```python
from build123d import *


with BuildPart() as f1:
    # F0 (on Front) → F1 (revolve)
    with BuildSketch(Plane.XZ):
        with BuildLine():
            Line((0, 201.6125), (0, 114.3))
            Line((0, 114.3), (0, 26.9875))
            ThreePointArc((0, 26.9875), (1.5875, 25.4), (3.175, 26.9875))
            Line((3.175, 26.9875), (3.175, 28.575))
            Line((3.175, 28.575), (2.159, 28.575))
            Line((2.159, 28.575), (2.159, 31.75))
            Line((2.159, 31.75), (3.175, 31.75))
            Line((3.175, 31.75), (3.175, 114.3))
            Line((3.175, 114.3), (3.175, 196.85))
            Line((3.175, 196.85), (2.159, 196.85))
            Line((2.159, 196.85), (2.159, 200.025))
            Line((2.159, 200.025), (3.175, 200.025))
            Line((3.175, 200.025), (3.175, 201.6125))
            ThreePointArc((3.175, 201.6125), (1.5875, 203.2), (0, 201.6125))
        make_face()
    revolve(axis=Axis((15.875, 0, 158.75), (0, 0, -1)))


solid = f1.part
```
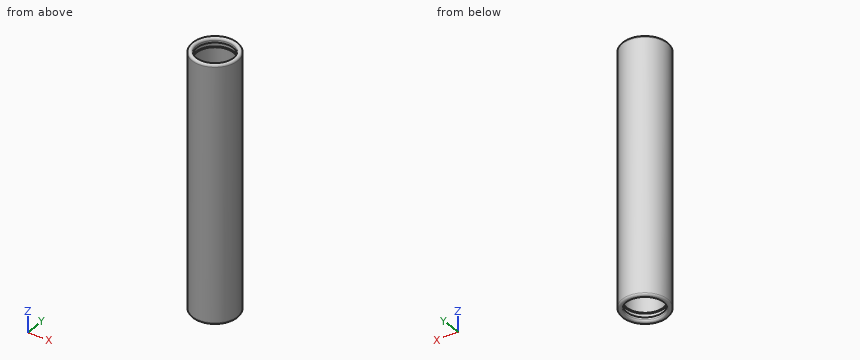
Check sheet for the modelled part. Datum: model origin and axes. Units: mm. Round coordinates to 2 decimals unless told otherwise and drop trailing zeros. Order: outer loops, then holes, each group sorted by start corner. A loop starts at its lowest first (then second) coordinate and runs counter-clockwise, first axis right, second up. Notation, with made-up numbers: (24, 18) - (35, 18) arc R11 ccw to (35, 39) - close; hole circle Ø8 at (4, 66.5). An arc over 180 degrees is marked (long way). Write item = value, one per line.
Q1. Thickness scan on line 1 along Z through (x, y) = (25, 10) (3 decimals); line 2 along Y through (x, z) = (15.5, 58.5); line 3 along Y through (x, z) = (27, 113). Record the ranges inside material, lowest first.
Computed:
line_1 = 25.588 to 28.575, 31.75 to 196.85, 200.025 to 203.012
line_2 = -15.87 to -12.69, 12.69 to 15.87
line_3 = -11.32 to -6.13, 6.13 to 11.32
Q2. Section check B-B (z = 88). Record the boundary of the cut face in (x, y) (3 decimals), and give its area (3 significant figures).
Computed:
outline = circle Ø31.75 at (15.875, 0); hole circle Ø25.4 at (15.875, 0)
area = 285 mm^2
Q3. Go/stop test with flat-tipped pins: pin 1 (12 mm diameter, centred on x = 9, y = 11.5, fed in from -Z); pin 2 (1.5 mm diameter, centred on y = -8, z = 75, fed in from +X); pin 3 (8 mm diameter, centred on x = 8.5, z = 84, fed in from -Y); pin 4 (1.5 mm diameter, centred on x = 5, z = 152.5, fed in from +Y). Record where each tip stops, or that it passes through.
Computed:
pin_1 = 25.4
pin_2 = 30
pin_3 = -15.51
pin_4 = 12.23
